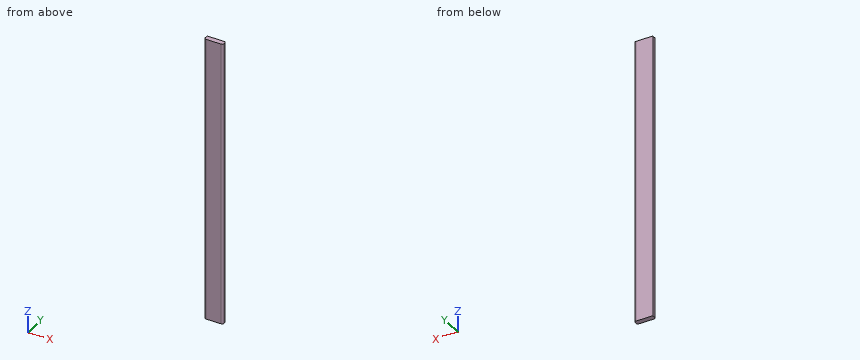
from build123d import *

# Parameters (mm, degrees)
F0_W     = 139.7
F0_H     = 38.1
F1_DEPTH = 2133.6
F2_R     = 12.7
F3_R     = 12.7
F4_R     = 12.7


with BuildPart() as f1:
    # F0 (on Top) → F1 (new body)
    with BuildSketch(Plane.XY):
        with Locations((-6.848779, -48.959874)):
            Rectangle(F0_W, F0_H)
    extrude(amount=F1_DEPTH)

    # F2
    f2_edges = [f1.edges().sort_by_distance(p)[0] for p in [
        (-76.698779, -68.009874, 1066.8),
    ]]
    fillet(f2_edges, radius=F2_R)

    # F3
    f3_edges = [f1.edges().sort_by_distance(p)[0] for p in [
        (63.001221, -68.009874, 1066.8),
    ]]
    fillet(f3_edges, radius=F3_R)

    # F4
    f4_edges = [f1.edges().sort_by_distance(p)[0] for p in [
        (63.001221, -29.909874, 1066.8),
    ]]
    fillet(f4_edges, radius=F4_R)


solid = f1.part
Verification items for the finished model (mm, model axes). Round coordinates to 2 decimals unless told otherwise and drop trailing zeros. Loops run counter-clockwise (first coordinate to the right, second up) from the corner with the lowest first, then second, coordinate; pieces in that order, holes last. Notation, with made-up numbers: (25.25, -9) - (49.25, -9) arc R35 cw to (49.25, 28) - close; hole circle Ø7 at (-37, -21). An arc over 180 degrees is marked (long way). Use one line per item in the form item = value.
1. Gauge pin test, flat ends, axial feed: pin 1 Ø8 at (y, z) = (-59.5, 321.5) entering from +X; pin 2 Ø1.5 at (y, z) = (-63.5, 1585.5) entering from -X. Record the tip position at first contact, or that the pin passes through.
A:
pin_1 = 63
pin_2 = -74.29
2. Scan lines: probe 1 along X at (y, z) = (-41, 1699); probe 2 along X at (y, z) = (-38.5, 1405.5); probe 3 along Y at (x, z) = (50.5, 96.5). Record each from-to range of solid material in increasing order.
A:
probe_1 = -76.7 to 62.9
probe_2 = -76.7 to 62.32
probe_3 = -68.01 to -29.91
3. Section check A-A on z = 1550. Record the cut outline in (x, y).
A:
outline = (-76.7, -55.31) arc R12.7 ccw to (-64, -68.01) - (50.3, -68.01) arc R12.7 ccw to (63, -55.31) - (63, -42.61) arc R12.7 ccw to (50.3, -29.91) - (-76.7, -29.91) - close
